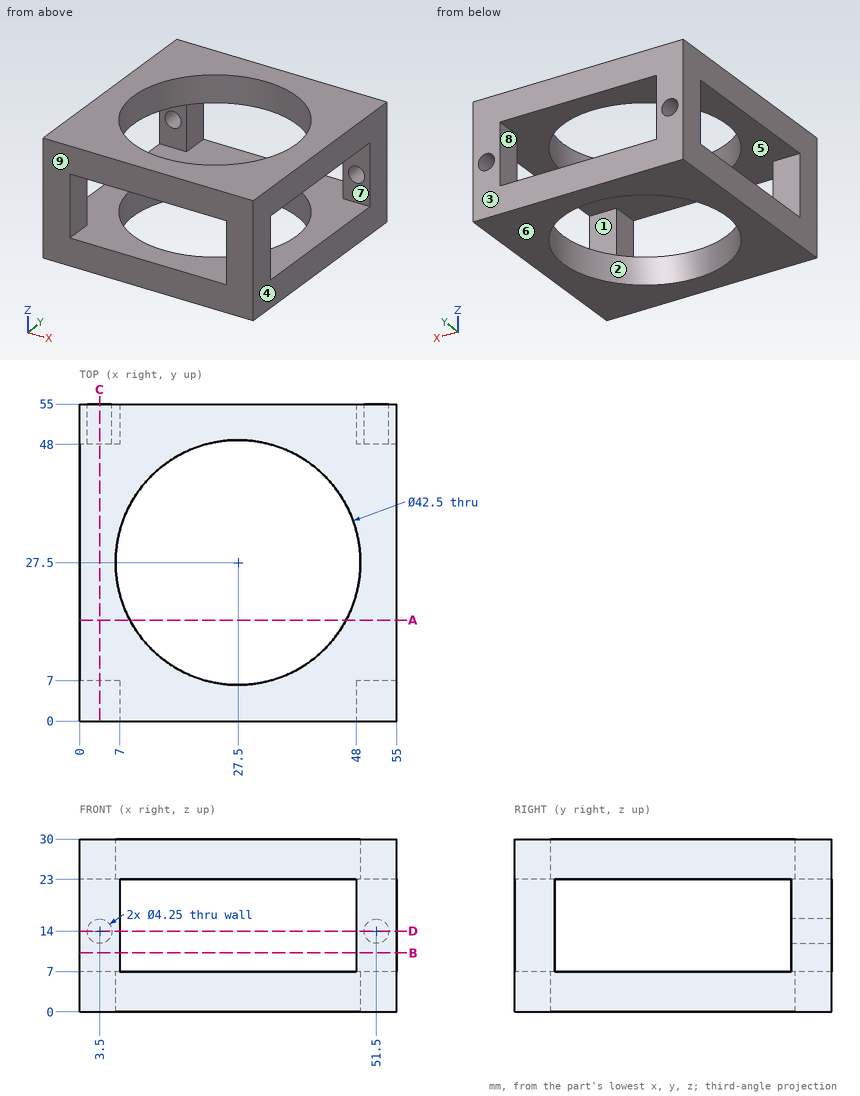
The drawing under review shows one solid part. Ordinate dimensions are in mm from its lowest x, y, z. A direction names the side the tool comes from. Coordinates: 2 decimals unless noted, no trailing zeros. Order: outer loops, then holes, each group sorted by start corner. A loop starts at its lowest first (then second) coordinate and runs counter-clockwise, first axis right, second up. Notation, with made-up numbers: (75, 89) -> (134, 89) arc R20 ccw to (134, 108) -> close; hole circle Ø2 at (9.25, 72). An arc over 180 degrees is marked (long way). Return JSON: item names as keys, results as strings.
1. The part is to be moulded in two halves that separate along Y. For the marked faces 1, 2, 3 and 4, say which applies: +Y half, -Y half, draft (parallel to the pull), parting line (faces both ways), or undercut.
Answer block:
{"face 1": "undercut", "face 2": "undercut", "face 3": "+Y half", "face 4": "draft"}
2. We need section A-A on y = 17.5. Write out the cut boundary in (x, z), and give its area (3 significant figures).
Answer block:
{"outline": "(0, 0) -> (8.75, 0) -> (8.75, 7) -> (0, 7) -> close; (0, 23) -> (8.75, 23) -> (8.75, 30) -> (0, 30) -> close; (46.25, 0) -> (55, 0) -> (55, 7) -> (46.25, 7) -> close; (46.25, 23) -> (55, 23) -> (55, 30) -> (46.25, 30) -> close", "area": "245 mm²"}
3. Machinability: for the marked faces 5, 6, 7, 8 and 9, which of the approach directions +Z, -Z, +X, -X, +Y, -Y give a long, thin tool a straight path to every point of the face, cutting with its end or side? Answer none if there is none.
Answer block:
{"face 5": "none", "face 6": "-Z, +X, -X, +Y, -Y", "face 7": "+X, -X", "face 8": "+Y, -Y", "face 9": "+Z, -Z, +X, -X, -Y"}
4. We need section D-D on z = 14. Write out the cut boundary in (x, y) (3 decimals), and give its area (4 significant figures).
Answer block:
{"outline": "(0, 0) -> (7, 0) -> (7, 7) -> (0, 7) -> close; (0, 48) -> (1.375, 48) -> (1.375, 55) -> (0, 55) -> close; (5.625, 48) -> (7, 48) -> (7, 55) -> (5.625, 55) -> close; (48, 0) -> (55, 0) -> (55, 7) -> (48, 7) -> close; (48, 48) -> (49.375, 48) -> (49.375, 55) -> (48, 55) -> close; (53.625, 48) -> (55, 48) -> (55, 55) -> (53.625, 55) -> close", "area": "136.5 mm²"}
5. We need section B-B on z = 10.25. Write out the cut boundary in (x, y), and give its area (3 significant figures).
Answer block:
{"outline": "(0, 0) -> (7, 0) -> (7, 7) -> (0, 7) -> close; (0, 48) -> (7, 48) -> (7, 55) -> (0, 55) -> close; (48, 0) -> (55, 0) -> (55, 7) -> (48, 7) -> close; (48, 48) -> (55, 48) -> (55, 55) -> (48, 55) -> close", "area": "196 mm²"}
6. For line 1 (X direction, y = 53.25, z = 14) (3 decimals); line 2 (X direction, y = 49, z = 11.5); line 3 (X direction, y = 27.5, z = 5.25), list the stretches that pass through material, from the lowest coordinate up. Write a range as from..to.
Answer block:
{"line 1": "0..1.375, 5.625..7, 48..49.375, 53.625..55", "line 2": "0..7, 48..55", "line 3": "0..6.25, 48.75..55"}
7. We need section C-C on x = 3.5. Write out the cut boundary in (y, z) (3 decimals).
Answer block:
{"outline": "(0, 0) -> (55, 0) -> (55, 11.875) -> (48, 11.875) -> (48, 7) -> (7, 7) -> (7, 23) -> (48, 23) -> (48, 16.125) -> (55, 16.125) -> (55, 30) -> (0, 30) -> close"}
